Geometry check sheet. Reference: the model listing, model coordinates, mm. A direction names the side the tool comes from. Round coordinates to 2 decimals unless told otherwise and drop trailing zeros. Order: outer loops, then holes, each group sorted by start corner. A loop starts at its lowest first (then second) coordinate and runs counter-clockwise, first axis right, second up. Notation, with made-up numbers: M 16.25,-13 L 64.25,-13 A22 cw 64.25,-2 Z; hole C 81.25,76 d8. An arc over 180 degrees is marked long. Answer as a JSON object with one key per item and string values. Group by question number.
Autodesk Inventor part; units mm, degrees
ref_plane "YZ Plane" through (0, 0, 0) normal (1, 0, 0) x (0, 1, 0)
ref_plane "XZ Plane" through (0, 0, 0) normal (0, 1, 0) x (-1, 0, 0)
ref_plane "XY Plane" through (0, 0, 0) normal (0, 0, 1) x (1, 0, 0)
sketch "Sketch1" plane through (0, 0, 0) normal (0, 0, 1) x (1, 0, 0)
  line L0 (73.279, 0) -> (73.279, 88.9)
  line L1 (0, 88.9) -> (0, 0)
  arc A0 (28.702, 76.2) -> (44.577, 76.2) centre (36.6395, 76.2) ccw
  line L2 (28.702, 76.2) -> (28.702, 88.9)
  line L3 (44.577, 76.2) -> (44.577, 88.9)
  line L4 (73.279, 88.9) -> (44.577, 88.9)
  line L5 (28.702, 88.9) -> (0, 88.9)
  line L6 (23.8252, 0) -> (49.4538, 0)
  line L7 (49.4538, 0) -> (49.4538, 25.4)
  line L8 (49.4538, 25.4) -> (23.8252, 25.4)
  line L9 (23.8252, 25.4) -> (23.8252, 0)
  line L10 (0, 25.4) -> (17.526, 0)
  line L11 (73.279, 25.4) -> (55.753, 0)
  line L12 (0, 0) -> (23.8252, 0)
  line L13 (49.4538, 0) -> (73.279, 0)
  dimension "d0" = 73.279
  dimension "d1" = 88.9
  dimension "d2" = 15.875
  dimension "d4" = 25.6286
  dimension "d5" = 63.5
  dimension "d6" = 23.8252
  dimension "d7" = 17.526
  dimension "d8" = 17.526
extrude "Extrusion1" add sketch "Sketch1" along normal blind 25.4 contours L11 L13 L7 L8 L9 L12 L10 L1 L5 L2 A0 L3 L4 L0
sketch "Sketch2" plane through (0, 0, 25.4) normal (0, 0, 1) x (1, 0, 0)
  circle A0 centre (36.6395, 61.9252) radius 3.2385
  line L0 (73.279, 25.4) -> (73.279, 88.9)
  line L1 (0, 88.9) -> (0, 25.4)
  line L2 (73.279, 88.9) -> (44.577, 88.9)
  point P0 (0, 0)
  dimension "d12" = 73.279
  dimension "d13" = 36.6395
  dimension "d14" = 6.477
  dimension "d15" = 26.9748
extrude "Extrusion2" cut sketch "Sketch2" against normal blind 14.2748
sketch "Sketch3" plane through (23.8252, 25.4, 0) normal (0, -1, 0) x (1, 0, 0)
  line L0 (0, 25.4) -> (25.6286, 25.4)
  line L1 (25.6286, 0) -> (25.6286, 25.4)
  point P0 (-23.8252, 0)
  point P1 (12.8143, 12.7)
  dimension "d18" = 12.7
  dimension "d19" = 12.8143
  dimension "d20" = 25.6286
hole "Hole1" at (36.6395, 25.4, 12.7) direction (0, 1, 0) diameter 7.7978 depth 19.05 tip angle 118
chamfer "Chamfer1" distance 1.524 angle 45 8 edges at (14.351, 88.9, 25.4) (0, 57.15, 25.4) (8.763, 12.7, 25.4) (20.6756, 0, 25.4) (52.6034, 0, 25.4) (64.516, 12.7, 25.4) (73.279, 57.15, 25.4) (58.928, 88.9, 25.4)
equation "\"d13\" = 0.5 * d12"
properties part number "Base" material "Stainless Steel"
1) Thickness scan on line 1 along X through (y, z) = (38.75, 12.7); line 2 along X through (y, z) = (83.5, 2); line 3 along Y through (x, z) = (35.5, 11.75). Record the ranges inside material, lowest first. Write a range as [from, to].
2) Sectioned sample at D-D (z = 20.5). Record the boundary of the cut face in (x, y) (1 decimal), then the cut area to 3 significant figures.
3) Release check for a two-part mould opening along X. For faces 1 (the flat face through (40, 25.4, 10)), 2 (the flat face through (0, 58, 12)), 3 (the flat face through (53, 0, 12)) record: +X half, -X half, draft (parallel to the pull), parting line (faces both ways), or undercut.
4) Go/stop test with flat-tipped pins: P1, Ø10, axis at x = 36.64, z = 12.7, coming from the +Y side; P2, Ø7.5, axis at x = 40.5, z = 10.5, coming from the -Y side; P3, Ø1, axis at y = 11, z = 10, coming from the -X side. Record where each tip stops, or that it passes through.
5) Sectioned sample at A-A (z = 3). Record the boundary of the cut face in (x, y) (1 decimal).
6) Sectioned sample at C-C (y = 74.5). Record the boundary of the cut face in (x, z) (3 decimals).
7) Sectioned sample at B-B (x = 47). Record the boundary of the cut face in (y, z), then the cut area to 3 significant figures.
8) Set-up check for faces 4 (the flat face through (28.702, 82, 13)), 5 (the cylindrical face through (35.47, 35.06, 8.98)), 6 (the flat face through (37, 62, 11.125)): record each of +Z, -Z, +X, -X, +Y, -Y from which the full face is reachable in a straight line by a thin tool's end or side.
Final values:
{
 "1": {"line 1": "x = [0, 32.74], [40.54, 73.28]", "line 2": "x = [0, 28.7], [44.58, 73.28]", "line 3": "y = [45.9, 58.89], [64.96, 68.34]"},
 "2": {"outline": "M 0,25.4 L 17.5,0 L 23.8,0 L 23.8,25.4 L 49.5,25.4 L 49.5,0 L 55.8,0 L 73.3,25.4 L 73.3,88.9 L 44.6,88.9 L 44.6,76.2 A7.9 cw 28.7,76.2 L 28.7,88.9 L 0,88.9 Z; hole C 36.6,61.9 d6.5", "area": "5,080 mm^2"},
 "3": {"face 1": "undercut", "face 2": "-X half", "face 3": "draft"},
 "4": {"P1": "stops at y = 70.04", "P2": "stops at y = 25.4", "P3": "stops at x = 9.59"},
 "5": {"outline": "M 0,25.4 L 17.5,0 L 23.8,0 L 23.8,25.4 L 49.5,25.4 L 49.5,0 L 55.8,0 L 73.3,25.4 L 73.3,88.9 L 44.6,88.9 L 44.6,76.2 A7.9 cw 28.7,76.2 L 28.7,88.9 L 0,88.9 Z"},
 "6": {"outline": "M 0,0 L 28.886,0 L 28.886,25.4 L 1.524,25.4 L 0,23.876 Z; M 44.393,0 L 73.279,0 L 73.279,23.876 L 71.755,25.4 L 44.393,25.4 Z"},
 "7": {"outline": "M 25.4,0 L 88.9,0 L 88.9,23.88 L 87.38,25.4 L 25.4,25.4 Z", "area": "1,610 mm^2"},
 "8": {"face 4": "+Z, -Z, +Y", "face 5": "-Y", "face 6": "+Z"}
}
